Job drawing, mm, ordinate dimensions from the low corner. One solid piece. A direction names the side the tool comes from. Give positions to 0.01 mm unless a question says otherwise; leave off trailing zeros. Order: outer loops, then holes, each group sorted by start corner. A loop starts at its lowest first (then second) coordinate and runs counter-clockwise, first axis right, second up.
Item 1: Two-plate mould, pull along X, no slides. Class the marked faces 1, 2 and 3: released by +X, released by -X, zero draft, split by the parting line, or undercut.
Item 2: Which spindle directions (+Z, -Z, +X, -X, +Y, -Y) get a long thin tool onto all of the face, cutting with end or side? Do the marked faces 4, 5 and 6. Say none if no direction does.
Item 3: Wall check: L1, parallel to Y at x = 6.5, z = 4.5; L2, parallel to Y at x = 50.8, z = 3; L3, parallel to X at y = 3, z = 2.25 (3 decimals). Give the ranges that are in metal, low to high.
Item 4: Band-saw the part on C-C on y = 28. Give the cut face in (x, z).
Item 5: Flat gauge pin, fed straight in: P1, Ø1.9, axis at y = 15.5, z = 3.5, coming from the +X side. Where does the tip first touch, or does it go through?
Item 6: Band-saw the part on A-A on x = 50.8. Give the cut face in (y, z), plus the area to 4 significant figures.
Item 7: Band-saw the part on B-B on y = 15.24. Give the cut face in (x, z) (3 decimals).
Item 8: Band-saw the part on D-D on z = 5.5. Give the cut face in (x, y) (3 decimals), plus the area to 3 significant figures.
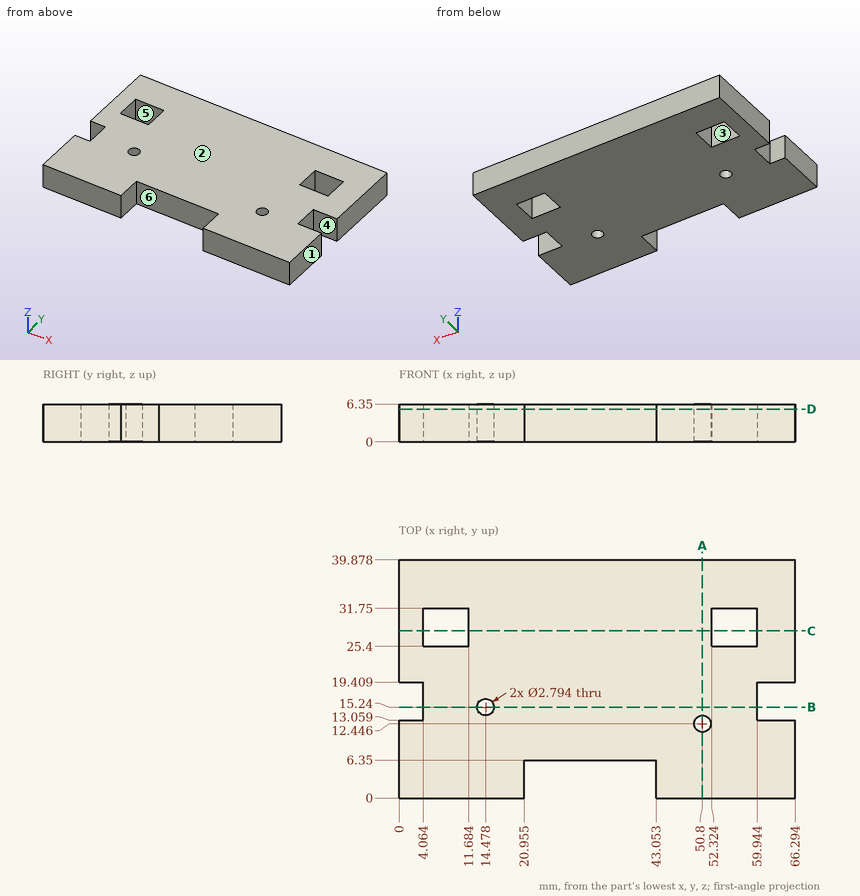
The answers:
1. face 1: released by +X
1. face 2: zero draft
1. face 3: undercut
2. face 4: +Z, -Z, +X
2. face 5: +Z, -Z
2. face 6: +Z, -Z, -Y
3. L1: y = 0 to 25.4, 31.75 to 39.88
3. L2: y = 0 to 11.05, 13.84 to 39.88
3. L3: x = 0 to 20.955, 43.053 to 66.294
4. outline: (0, 0) - (4.06, 0) - (4.06, 6.35) - (0, 6.35) - close; (11.68, 0) - (52.32, 0) - (52.32, 6.35) - (11.68, 6.35) - close; (59.94, 0) - (66.29, 0) - (66.29, 6.35) - (59.94, 6.35) - close
5. P1: stops at x = 59.94
6. outline: (0, 0) - (11.05, 0) - (11.05, 6.35) - (0, 6.35) - close; (13.84, 0) - (39.88, 0) - (39.88, 6.35) - (13.84, 6.35) - close
6. area: 235.5 mm2
7. outline: (4.064, 0) - (13.081, 0) - (13.081, 6.35) - (4.064, 6.35) - close; (15.875, 0) - (59.944, 0) - (59.944, 6.35) - (15.875, 6.35) - close
8. outline: (0, 0) - (20.955, 0) - (20.955, 6.35) - (43.053, 6.35) - (43.053, 0) - (66.294, 0) - (66.294, 13.059) - (59.944, 13.059) - (59.944, 19.409) - (66.294, 19.409) - (66.294, 39.878) - (0, 39.878) - (0, 19.409) - (4.064, 19.409) - (4.064, 13.059) - (0, 13.059) - close; hole (4.064, 25.4) - (11.684, 25.4) - (11.684, 31.75) - (4.064, 31.75) - close; hole circle Ø2.794 at (14.478, 15.24); hole circle Ø2.794 at (50.8, 12.446); hole (52.324, 25.4) - (59.944, 25.4) - (59.944, 31.75) - (52.324, 31.75) - close
8. area: 2,330 mm2
